Build history of the part. All positions in model axes, mm. Face numbers are marked on the shaded views. A direction names the side the tool comes from. Coordinates: 2 decimals unless noted, no trailing zeros. Order: outer loops, then holes, each group sorted by start corner. A loop starts at its lowest first (then second) coordinate and runs counter-clockwise, first axis right, second up. Notation, with made-up numbers: (52, -18) - (60, -18) arc R30 ccw to (60, 20) - close; hole circle Ø9 at (1.25, 5). An arc over 180 degrees is marked (long way). Return JSON: item names as keys, results as strings.
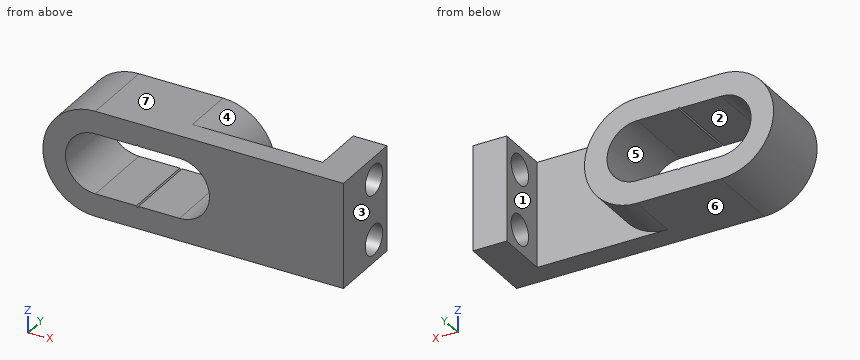
Autodesk Inventor part; units mm, degrees
ref_plane "YZ Plane" through (0, 0, 0) normal (1, 0, 0) x (0, 1, 0)
ref_plane "XZ Plane" through (0, 0, 0) normal (0, 1, 0) x (-1, 0, 0)
ref_plane "XY Plane" through (0, 0, 0) normal (0, 0, 1) x (1, 0, 0)
sketch "Sketch1" plane through (0, 0, 0) normal (0, 1, 0) x (-1, 0, 0)
  arc A0 (0, 4) -> (0, -4) centre (0, 0) ccw
  arc A1 (11.1938, -4) -> (11.1938, 4) centre (11.1938, 0) ccw
  line L0 (11.1938, -4) -> (0, -4)
  line L1 (11.1938, 4) -> (0, 4)
  line L2 (11.1938, -7) -> (0, -7)
  line L3 (0, 7) -> (11.1938, 7)
  arc A2 (5.5969, 4.2041) -> (5.4492, 4) centre (11.1938, 0) ccw
  arc A3 (5.7446, 4) -> (5.5969, 4.2041) centre (0, 0) ccw
  arc A4 (5.4492, -4) -> (5.5969, -4.2041) centre (11.1938, 0) ccw
  arc A5 (11.1938, -7) -> (11.1938, 7) centre (11.1938, 0) ccw
  arc A6 (0, 7) -> (0, -7) centre (0, 0) ccw
  arc A7 (5.5969, -4.2041) -> (5.7446, -4) centre (0, 0) ccw
  dimension "d0" = 8
  dimension "d1" = 8
extrude "Extrusion1" add sketch "Sketch1" along normal blind 10
sketch "Sketch2" plane through (0, 0, 0) normal (0, -1, 0) x (1, 0, 0)
  arc A0 (0, -7) -> (0, 7) centre (0, 0) ccw
  arc A1 (0, -4) -> (0, 4) centre (0, 0) ccw
  line L0 (0, -7) -> (0, -4)
  line L1 (0, 4) -> (0, 7)
  line L2 (0, -7) -> (-11.1938, -7)
  line L3 (0, -7) -> (17.35, -7)
  arc A2 (0, -7) -> (0, 7) centre (0, 0) ccw
  line L4 (0, 7) -> (17.35, 7)
  line L5 (17.35, 7) -> (17.35, -7)
  dimension "d6" = 17.35
extrude "Extrusion2" add sketch "Sketch2" against normal blind 3 contours A0 L4 L5 L3
sketch "Sketch3" plane through (17.35, 0, 7) normal (1, 0, 0) x (0, 0, -1)
  line L0 (14, 10) -> (0, 10)
  line L1 (0, 0) -> (14, 0)
  line L2 (14, 0) -> (14, 10)
  line L3 (14, 10) -> (0, 10)
  line L4 (0, 10) -> (0, 0)
  point P0 (7, 0)
extrude "Extrusion3" add sketch "Sketch3" along normal blind 4.5
sketch "Sketch4" plane through (21.85, 0, 7) normal (1, 0, 0) x (0, 0, -1)
  circle A0 centre (3, 7) radius 2
  circle A1 centre (11, 7) radius 2
  line L0 (14, 10) -> (0, 10)
  line L1 (0, 10) -> (0, 0)
  line L2 (14, 0) -> (14, 10)
  point P0 (7, 0)
  dimension "d11" = 4
  dimension "d12" = 4
  dimension "d13" = 3
  dimension "d14" = 3
  dimension "d15" = 3
  dimension "d16" = 3
extrude "Extrusion4" cut sketch "Sketch4" against normal blind 5
properties part number "bedtiedown2"
1. Mould opens along Z. For the marked faces 5, 6 and 7 say: pulls with the +Z half, pulls with the -Z half, needs draft (parallel to the pull), parting line crosses it, or undercut.
Check values:
{"face 5": "undercut", "face 6": "pulls with the -Z half", "face 7": "pulls with the +Z half"}
2. Tool access for the marked faces 1, 2, 3 and 4: list every direction of +Z, -Z, +X, -X, +Y, -Y with a clear straight run to the whole face (end or side of a thin tool).
Check values:
{"face 1": "+Z, -Z, +Y", "face 2": "+Y, -Y", "face 3": "+Z, -Z, +X, +Y, -Y", "face 4": "+Y"}
3. Cut at B-B on z = 0. Give the cut face in (x, y), plus the area to 3 significant figures.
Check values:
{"outline": "(-18.19, 0) - (-15.19, 0) - (-15.19, 10) - (-18.19, 10) - close; (4, 0) - (21.85, 0) - (21.85, 10) - (17.35, 10) - (17.35, 3) - (7, 3) - (7, 10) - (4, 10) - close", "area": "136 mm²"}
4. Cut at A-A on y = 3.75. Give the cut face in (x, z).
Check values:
{"outline": "(-11.19, -7) - (0, -7) arc R7 ccw to (0, 7) - (-11.19, 7) arc R7 ccw to start; (17.35, -7) - (21.85, -7) - (21.85, 7) - (17.35, 7) - close; hole (-11.19, -4) - (-5.74, -4) arc R7.15 ccw to (-5.6, -4.2) arc R6.85 ccw to (-5.45, -4) - (0, -4) arc R4 ccw to (0, 4) - (-5.45, 4) arc R7.15 ccw to (-5.6, 4.2) arc R6.85 ccw to (-5.74, 4) - (-11.19, 4) arc R4 ccw to start"}
5. Drop flat-ended pins along their axis: pin 1 (3.5 mm diameter, centred on y = 7, z = -4, fed in from -X); pin 2 (7 mm diameter, centred on x = 10, z = -3.5, fed in from +Y); pin 3 (1 mm diameter, centred on y = 5, z = -3.5, fed in from -X). Give the stop position or say it passes through.
Check values:
{"pin 1": "x = -17.82", "pin 2": "y = 3", "pin 3": "x = -17.52"}
6. Cut at C-C on x = -6.5. Give the cut face in (y, z).
Check values:
{"outline": "(0, -7) - (10, -7) - (10, -4) - (0, -4) - close; (0, 4) - (10, 4) - (10, 7) - (0, 7) - close"}
7. Probe L1, parallel to X at y = 8.5, z = 2.5; L2, parallel to Y at x = 19.85, z = -4; L3, parallel to X at y = 5.25, z = 5.75. List the from-to ranges inside material, lowest first.
Check values:
{"L1": "-17.73 to -14.32, 3.12 to 6.54, 17.35 to 21.85", "L2": "0 to 5, 9 to 10", "L3": "-15.19 to 3.99, 17.35 to 21.85"}
8. Cut at D-D on y = 5.75. Give the cut face in (x, z).
Check values:
{"outline": "(-11.19, -7) - (0, -7) arc R7 ccw to (0, 7) - (-11.19, 7) arc R7 ccw to start; (17.35, -7) - (21.85, -7) - (21.85, -5.56) - (17.35, -5.56) - close; (17.35, -2.44) - (21.85, -2.44) - (21.85, 2.44) - (17.35, 2.44) - close; (17.35, 5.56) - (21.85, 5.56) - (21.85, 7) - (17.35, 7) - close; hole (-11.19, -4) - (-5.74, -4) arc R7.15 ccw to (-5.6, -4.2) arc R6.85 ccw to (-5.45, -4) - (0, -4) arc R4 ccw to (0, 4) - (-5.45, 4) arc R7.15 ccw to (-5.6, 4.2) arc R6.85 ccw to (-5.74, 4) - (-11.19, 4) arc R4 ccw to start"}
